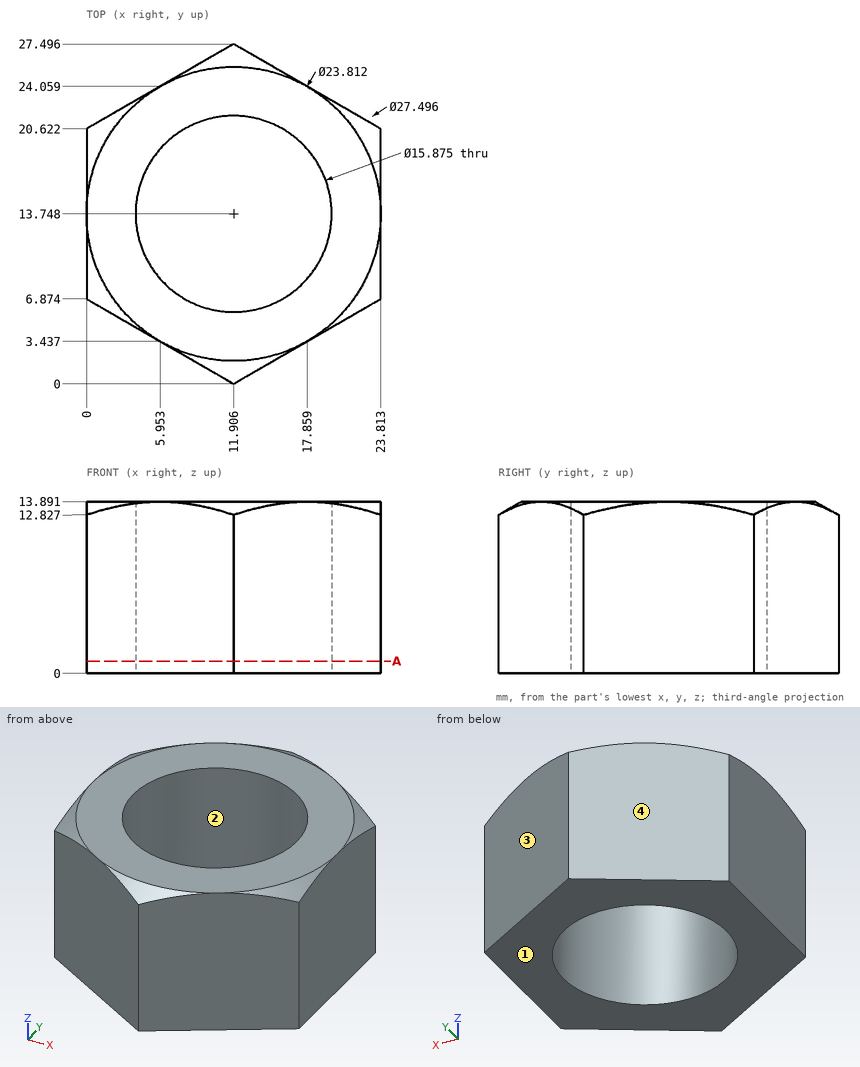
The figure shows three views and two pictorial views of one solid part (mm, origin at its lowest corner). Answer the questions. Round coordinates to 2 decimals unless told otherwise and drop trailing zeros. Order: outer loops, then holes, each group sorted by start corner. A loop starts at its lowest first (then second) coordinate and runs counter-clockwise, first axis right, second up. Notation, with made-up numbers: M 75,22.25 L 130,22.25 A27 cw 130,48.25 Z; hole C 46.5,6 d9. An arc over 180 degrees is marked long. Put each result on its own line as item: value. Start each with the question number.
Q1. A flat-ended cylindrical pin translates along its axis: pin 1 (1.5 mm diameter, centred on y = 22.5, z = 10, fed in from -X) (1 decimal). Find the tip coordinate at first contact, or state that the pin passes through.
Q2. Straight lines are drawn through the part: L1, parallel to X at y = 13.75, z = 11.5; L2, parallel to Y at x = 17, z = 5.25 (1 decimal); L3, parallel to X at y = 18.75, z = 6 (1 decimal). For each, find the intervals that lie inside material, in ascending order. Write a range as [from, to].
Q3. For a pull along X with two mould halves and no side action, classify the marked faces 1, 2, 3 and 4 as pulls with the +X half, pulls with the -X half, needs draft (parallel to the pull), parting line crosses it, or undercut.
Q4. Section A-A, the plane z = 1 is taken. Write down the section's boundary in (x, y) (1 decimal), and give its area (3 significant figures).
Findings below:
1. pin 1: stops at x = 2
2. L1: x = [0, 3.97], [19.84, 23.81]
2. L2: y = [2.9, 7.7], [19.8, 24.6]
2. L3: x = [0, 5.7], [18.1, 23.8]
3. face 1: needs draft
3. face 2: undercut
3. face 3: pulls with the +X half
3. face 4: pulls with the -X half
4. outline: M 0,6.9 L 11.9,0 L 23.8,6.9 L 23.8,20.6 L 11.9,27.5 L 0,20.6 Z; hole C 11.9,13.7 d15.9
4. area: 293 mm^2
